```python
from build123d import *

# Parameters (mm, degrees)
SKETCH1_W                                           = 17.5
SKETCH1_H                                           = 23.5
SKETCH1_R                                           = 3.5
BOSS_EXTRUDE1_DEPTH                                 = 3
CSK_FOR_M2_COUNTERSUNK_FLAT_HEAD_SCREW1_D           = 2.4
CSK_FOR_M2_COUNTERSUNK_FLAT_HEAD_SCREW1_CSINK_D     = 4.4
CSK_FOR_M2_COUNTERSUNK_FLAT_HEAD_SCREW1_CSINK_ANGLE = 90
TAP_DRILL_FOR_M3_TAP1_D                             = 2.5
TAP_DRILL_FOR_M3_TAP1_DEPTH                         = 6
TAP_DRILL_FOR_M3_TAP1_TIP                           = 0.751075774


with BuildPart() as part:
    # Sketch1 → Boss-Extrude1 (new, symmetric)
    with BuildSketch(Plane.XY):
        Rectangle(SKETCH1_W, SKETCH1_H)
        with Locations((0, -1.53)):
            Circle(SKETCH1_R, mode=Mode.SUBTRACT)
    extrude(amount=BOSS_EXTRUDE1_DEPTH, both=True)

    # CSK for M2 Countersunk Flat Head Screw1 (through all)
    with Locations(Plane.XY.offset(3)):
        with Locations((0, -7.53), (-5.196152423, 1.47), (5.196152423, 1.47)):
            CounterSinkHole(CSK_FOR_M2_COUNTERSUNK_FLAT_HEAD_SCREW1_D / 2, CSK_FOR_M2_COUNTERSUNK_FLAT_HEAD_SCREW1_CSINK_D / 2, counter_sink_angle=CSK_FOR_M2_COUNTERSUNK_FLAT_HEAD_SCREW1_CSINK_ANGLE)

    # Tap Drill for M3 Tap1
    with Locations(Plane(origin=(0, 11.75, 0), x_dir=(1, 0, 0), z_dir=(0, 1, 0))):
        with Locations((-5, 0), (5, 0)):
            Hole(TAP_DRILL_FOR_M3_TAP1_D / 2, depth=TAP_DRILL_FOR_M3_TAP1_DEPTH)
            with Locations((0, 0, -(TAP_DRILL_FOR_M3_TAP1_DEPTH + TAP_DRILL_FOR_M3_TAP1_TIP / 2))):  # 118° drill point
                Cone(0, TAP_DRILL_FOR_M3_TAP1_D / 2, TAP_DRILL_FOR_M3_TAP1_TIP, mode=Mode.SUBTRACT)


solid = part.part
```
Input: part model. Units: mm. Frame: model coordinates. A direction names the side the tool comes from. Coordinates: 2 decimals unless noted, no trailing zeros. Write each loop counter-clockwise with the first axis right and the second up, starting at its lowest first coordinate (ties: lowest second). Pieces come first, ordered by that corner, then holes.
1) Set-up query: faces 1 (the cylindrical face through (-3.75, 8.71, -0.05)), 2 (the cylindrical face through (-0.759, -4.947, -0.042)). Return all of +Z, -Z, +X, -X, +Y, -Y with unobstructed straight access to the full face (end or side cutting, diameter ignored); none if empty.
2) Material intervals for line 1 along X through (y, z) = (7, -0.05); line 2 along Y through (x, z) = (0, 0.7); line 3 along Z through (x, y) = (-5, 10.3), sorted ascending.
3) Section C-C on y = -1.53. Output: boundary loops of the cut face in (x, z), and give its area (3 significant figures).
4) Pin query (flat end, axial travel): pin 1 Ø3 at (x, y) = (-5.5, 1.5) entering from +Z; pin 2 Ø4 at (x, y) = (5.2, 1.47) entering from +Z; pin 3 Ø1 at (x, z) = (4.5, 0) entering from +Y. Return the tip coordinate at first contact, or that it passes through.
5) Section A-A on x = 0. Output: boundary loops of the cut face in (y, z), and give its area (3 significant figures).
6) Section B-B on z = -1.5. Output: boundary loops of the cut face in (x, y).
7) Section D-D on x = -2.5. Output: boundary loops of the cut face in (y, z), and give its area (3 significant figures).
8) Mould query, pull axis X, two halves, no side actions, for faces 3 (the flat face through (8.75, 0, 0)), 4 (the flat face through (0, 11.75, 0)), 5 (the cylindrical face through (6.08, 2.28, -0.54)). Classes: pulls with the +X half, pulls with the -X half, needs draft (parallel to the pull), parting line crosses it, or undercut.
Check result:
1. face 1: +Y
1. face 2: +Z, -Z
2. line 1: x = -8.75 to -6.25, -3.75 to 3.75, 6.25 to 8.75
2. line 2: y = -11.75 to -8.73, -6.33 to -5.03, 1.97 to 11.75
2. line 3: z = -3 to -1.25, 1.25 to 3
3. outline: (-8.75, -3) - (-3.5, -3) - (-3.5, 3) - (-8.75, 3) - close; (3.5, -3) - (8.75, -3) - (8.75, 3) - (3.5, 3) - close
3. area: 63.0 mm2
4. pin 1: stops at z = 2.61
4. pin 2: stops at z = 2.8
4. pin 3: stops at y = 5.6
5. outline: (-11.75, -3) - (-8.73, -3) - (-8.73, 2) - (-9.73, 3) - (-11.75, 3) - close; (-6.33, -3) - (-5.03, -3) - (-5.03, 3) - (-5.33, 3) - (-6.33, 2) - close; (1.97, -3) - (11.75, -3) - (11.75, 3) - (1.97, 3) - close
5. area: 83.6 mm2
6. outline: (-8.75, -11.75) - (8.75, -11.75) - (8.75, 11.75) - (-8.75, 11.75) - close; hole circle Ø2.4 at (-5.2, 1.47); hole circle Ø7 at (0, -1.53); hole circle Ø2.4 at (0, -7.53); hole circle Ø2.4 at (5.2, 1.47)
7. outline: (-11.75, -3) - (-3.98, -3) - (-3.98, 3) - (-11.75, 3) - close; (0.92, -3) - (11.75, -3) - (11.75, 3) - (0.92, 3) - close
7. area: 112 mm2
8. face 3: pulls with the +X half
8. face 4: needs draft
8. face 5: undercut
